```python
from build123d import *

# Parameters (mm, degrees)
SKETCH1_R               = 76.2
BOSS_EXTRUDE1_DEPTH     = 101.6
SKETCH2_R               = 63.5
CUT_EXTRUDE1_DEPTH      = 25.4
SKETCH3_R               = 63.5
SKETCH3_R_2             = 50.8
BOSS_EXTRUDE2_DEPTH     = 12.7
SKETCH4_R               = 50.8
CUT_EXTRUDE2_DEPTH      = 102.6
CUT_EXTRUDE3_DEPTH      = 102.6
SKETCH6_W               = 63.5
SKETCH6_H               = 5.08
BOSS_EXTRUDE4_DEPTH     = 5.08
LPATTERN1_COUNT         = 2
LPATTERN1_PITCH         = 10.16
MIRROR1_COPY_1_SKETCH_W = 63.5
MIRROR1_COPY_1_SKETCH_H = 5.08
MIRROR1_COPY_1_DEPTH    = 5.08


with BuildPart() as part:
    # Sketch1 → Boss-Extrude1 (new body)
    with BuildSketch(Plane.XY):
        Circle(SKETCH1_R)
    extrude(amount=BOSS_EXTRUDE1_DEPTH)

    # Sketch2 → Cut-Extrude1 (cut)
    with BuildSketch(Plane.XY.offset(101.6)):
        Circle(SKETCH2_R)
    extrude(amount=-CUT_EXTRUDE1_DEPTH, mode=Mode.SUBTRACT)

    # Sketch3 → Boss-Extrude2 (add)
    with BuildSketch(Plane.XY.offset(101.6)):
        Circle(SKETCH3_R)
        Circle(SKETCH3_R_2, mode=Mode.SUBTRACT)
    extrude(amount=-BOSS_EXTRUDE2_DEPTH)

    # Sketch4 → Cut-Extrude2 (cut, through all)
    with BuildSketch(Plane(origin=(0, 0, 0), x_dir=(-1, 0, 0), z_dir=(0, 0, -1))):
        Circle(SKETCH4_R)
    extrude(amount=-CUT_EXTRUDE2_DEPTH, mode=Mode.SUBTRACT)

    # Sketch5 → Cut-Extrude3 (cut, through all)
    with BuildSketch(Plane.XY.offset(101.6)):
        with BuildLine():
            Line((0, 76.2), (0, -76.2))
            ThreePointArc((0, -76.2), (76.2, 0), (0, 76.2))
        make_face()
    extrude(amount=-CUT_EXTRUDE3_DEPTH, mode=Mode.SUBTRACT)

    # Sketch6 → Boss-Extrude4 (add)
    with BuildSketch(Plane(origin=(0, 0, 0), x_dir=(0, 0, -1), z_dir=(1, 0, 0))):
        with Locations((-31.75, -58.42)):
            Rectangle(SKETCH6_W, SKETCH6_H)
    boss_extrude4 = extrude(amount=BOSS_EXTRUDE4_DEPTH)

    # LPattern1: Boss-Extrude4 ×2
    with Locations(*[(0, -i * LPATTERN1_PITCH, 0) for i in range(1, LPATTERN1_COUNT)]):
        add(boss_extrude4)

    # Mirror1: Boss-Extrude4 across plane
    add(boss_extrude4.mirror(Plane.ZX))

    # Mirror1 copy 1 sketch → Mirror1 copy 1 (add)
    with BuildSketch(Plane(origin=(0, 10.16, 0), x_dir=(0, 0, -1), z_dir=(1, 0, 0))):
        with Locations((-31.75, 58.42)):
            Rectangle(MIRROR1_COPY_1_SKETCH_W, MIRROR1_COPY_1_SKETCH_H)
    extrude(amount=MIRROR1_COPY_1_DEPTH)


solid = part.part
```
CAD build for the part. Positions are in the model's coordinates, mm. A direction names the side the tool comes from. Coordinates: 2 decimals unless noted, no trailing zeros. Order: outer loops, then holes, each group sorted by start corner. A loop starts at its lowest first (then second) coordinate and runs counter-clockwise, first axis right, second up. Notation, with made-up numbers: (77.25, 60) - (95.25, 60) arc R5 ccw to (95.25, 64) - close; hole circle Ø2 at (37, -4.5). An arc over 180 degrees is marked (long way). Answer in a Markdown table with one row per item.
1. Pull direction Y, two halves, no side cores. Call faces 4 (the face through (5.08, -58, 32)), 5 (the face through (3, -60.96, 32)): +Y half, -Y half, draft (parallel to the pull), parting line (faces both ways), or undercut.
Answer:
| item | result |
|---|---|
| face 4 | draft |
| face 5 | undercut |
2. 3-axis set-ups, long thin cutter, end or side, ignore diameter. For faces 1 (the face through (3, 60.96, 32)), 2 (the face through (3, -69, 63.5)), 3 (the face through (-51, 5, 88.9)): which of +Z, -Z, +X, -X, +Y, -Y reach the whole face in a straight line?
Answer:
| item | result |
|---|---|
| face 1 | +Z, -Z, +X |
| face 2 | +Z, +X, +Y, -Y |
| face 3 | +X |
3. Slice it at A-A, the plane y = 0. List the corners of the cut face in (x, z).
Answer:
| item | result |
|---|---|
| outline | (-76.2, 0) - (-50.8, 0) - (-50.8, 76.2) - (-63.5, 76.2) - (-63.5, 88.9) - (-50.8, 88.9) - (-50.8, 101.6) - (-76.2, 101.6) - close |
4. Slice it at B-B, the plane x = -44. List the corners of the cut face in (y, z), then the cut area to 3 significant figures.
Answer:
| item | result |
|---|---|
| outline | (-62.21, 0) - (-25.39, 0) - (-25.39, 76.2) - (-45.78, 76.2) - (-45.78, 88.9) - (-25.39, 88.9) - (-25.39, 101.6) - (-62.21, 101.6) - close; (25.39, 0) - (62.21, 0) - (62.21, 101.6) - (25.39, 101.6) - (25.39, 88.9) - (45.78, 88.9) - (45.78, 76.2) - (25.39, 76.2) - close |
| area | 6,960 mm² |
5. Slice it at C-C, the plane z = 47.5. List the corners of the cut face in (x, y).
Answer:
| item | result |
|---|---|
| outline | (0, -76.2) - (0, -71.12) - (5.08, -71.12) - (5.08, -66.04) - (0, -66.04) - (0, -60.96) - (5.08, -60.96) - (5.08, -55.88) - (0, -55.88) - (0, -50.8) arc R50.8 cw to (0, 50.8) - (0, 55.88) - (5.08, 55.88) - (5.08, 60.96) - (0, 60.96) - (0, 66.04) - (5.08, 66.04) - (5.08, 71.12) - (0, 71.12) - (0, 76.2) arc R76.2 ccw to start |
6. Drill centre lines: L1, parallel to Z at x = -16, y = 49; L2, parallel to Y at x = -43, z = 9; L3, parallel to Y at x = -28, z = 81.5. Where is each one in solid material? Low to high. Write a range as from..to.
Answer:
| item | result |
|---|---|
| L1 | 0..76.2, 88.9..101.6 |
| L2 | -62.91..-27.05, 27.05..62.91 |
| L3 | -70.87..-56.99, 56.99..70.87 |
7. Slice it at D-D, the plane x = -60. List the corners of the cut face in (y, z).
Answer:
| item | result |
|---|---|
| outline | (-46.97, 0) - (46.97, 0) - (46.97, 101.6) - (-46.97, 101.6) - close; hole (-20.79, 76.2) - (20.79, 76.2) - (20.79, 88.9) - (-20.79, 88.9) - close |
8. Flat gauge pins, fed straight in: P1, Ø6, axis at x = -43.5, z = 39, coming from the -Y side; P2, Ø1.5, axis at y = -9, z = 86.5, coming from the -X side; P3, Ø8, axis at x = -34.5, z = 11.5, coming from the -Y side; P4, Ø19, axis at x = -38, y = -8.5, coming from the -Z side. Where does each tip first touch, or does it go through?
Answer:
| item | result |
|---|---|
| P1 | y = -64.55 |
| P2 | x = -75.75 |
| P3 | y = -69.83 |
| P4 | through |
